Here's how the part is built. I have some questions about the finished solid (model axes, mm). Face numbers are marked on the shaded views. A direction names the side the tool comes from. Coordinates: 2 decimals unless noted, no trailing zeros. Write each loop counter-clockwise with the first axis right and the second up, starting at its lowest first coordinate (ties: lowest second). Pieces come first, ordered by that corner, then holes. Notation, with made-up numbers: (58.25, -15) - (100.25, -15) arc R34 ccw to (100.25, 17) - close; hole circle Ø11 at (10.5, 59). An arc over 180 degrees is marked (long way). Answer in a Markdown table with one row per item. Add a question column.
Item 1: Imagine slicing it at D-D (z = -7.62). Please give me the cut outline in (x, y).
Item 2: We'd pull the mould along Y, two halves only. Please class the marked faces 1, 2, 3 and 4: +Y half, -Y half, draft (parallel to the pull), parting line (faces both ways), or undercut.
Item 3: Imagine slicing it at B-B (y = 17.25). Please give me the cut outline in (x, z), plus the area to 3 significant figures.
Item 4: I'm going to push flat-ended pins straight in: pin 1 (4 mm diameter, centred on y = 20.5, z = -2.5, fed in from -X); pin 2 (3.5 mm diameter, centred on y = 13.5, z = -3.5, fed in from +X); pin 3 (2 mm diameter, centred on y = 4.5, z = -8.5, fed in from +X). Where does each tip first touch, or does it pass through?
Item 5: Which directions (+Z, -Z, +X, -X, +Y, -Y) give clear straight access to the entire face, cutting with the end or side of a thin tool? Please do the marked faces 5, 6 and 7.
Item 6: If I drill on probe 1 along Y at (x, z) = (-22.5, -8.5); probe 2 along X at (y, z) = (10, -11.5); probe 3 along Y at (x, z) = (-20.5, -7.25), over which ranges is the centre line in solid material (lowest first)? Write a range as from..to.
Item 7: Imagine slicing it at A-A (z = -4.5). Please give me the cut outline in (x, y).
Item 8: Imagine slicing it at C-C (x = -32.5). Please give me the cut outline in (y, z).
Autodesk Inventor part; units mm, degrees
ref_plane "YZ Plane" through (0, 0, 0) normal (1, 0, 0) x (0, 1, 0)
ref_plane "XZ Plane" through (0, 0, 0) normal (0, 1, 0) x (-1, 0, 0)
ref_plane "XY Plane" through (0, 0, 0) normal (0, 0, 1) x (1, 0, 0)
sketch "Sketch1" plane through (0, 0, 0) normal (0, 0, 1) x (1, 0, 0)
  line L0 (-18.3846, 28.5) -> (-18.3846, 22)
  line L1 (-18.3846, 22) -> (-22.3846, 18)
  line L2 (-22.3846, 18) -> (-22.3846, 7)
  line L3 (-22.3846, 7) -> (-18.3846, 3)
  line L4 (-18.3846, 3) -> (-18.3846, -3.5)
  line L5 (-18.3846, 28.5) -> (-31.1346, 28.5)
  line L6 (-31.1346, 28.5) -> (-31.1346, -3.5)
  line L7 (-31.1346, -3.5) -> (-18.3846, -3.5)
  line L8 (-22.3846, 7) -> (-23.3846, 7)
  line L9 (-23.3846, 7) -> (-23.3846, 18)
  line L10 (-23.3846, 18) -> (-22.3846, 18)
  line L11 (-31.1346, 11.0301) -> (-37.4846, 11.0301) construction
  point P0 (0, 0)
  dimension "d0" = 1
  dimension "d1" = 6.35
  dimension "d2" = 8.75
  dimension "d13" = 135
  dimension "d14" = 135
  dimension "d15" = 11
  dimension "d16" = 12.75
  dimension "d17" = 32
extrude "Extrusion1" add sketch "Sketch1" against normal blind 12 contours L0 L1 L10 L9 L8 L3 L4 L7 L6 L5
sketch "Sketch3" plane through (-31.1346, -3.5, 0) normal (-1, 0, 0) x (0, 0, 1)
  line L0 (0, 32) -> (0, 0)
  line L1 (0, 32) -> (-12, 32)
  line L2 (-12, 0) -> (-12, 32)
  line L3 (0, 0) -> (-12, 0)
  circle A0 centre (-7.62, 11.25) radius 1.27
  circle A1 centre (-7.62, 20.75) radius 1.27
  line L4 (-12, 21.5) -> (-12, 10.5) construction
  line L5 (-12, 16) -> (0, 16) construction
  point P0 (0, 3.5)
  dimension "d8" = 2.54
  dimension "d9" = 9.5
  dimension "d10" = 7.62
extrude "Extrusion3" add sketch "Sketch3" along normal blind 5 contours A0 | A1
properties part number "Limit Adapter"
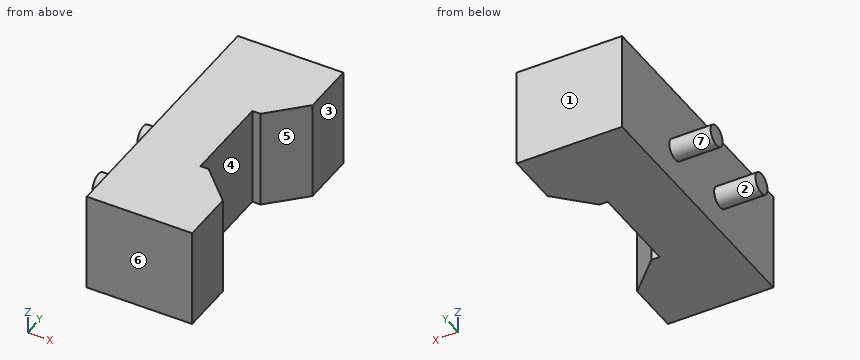
Here are the results:
| question | item | result |
|---|---|---|
| 1 | outline | (-36.13, 6.48) - (-31.13, 6.48) - (-31.13, -3.5) - (-18.38, -3.5) - (-18.38, 3) - (-22.38, 7) - (-23.38, 7) - (-23.38, 18) - (-22.38, 18) - (-18.38, 22) - (-18.38, 28.5) - (-31.13, 28.5) - (-31.13, 18.52) - (-36.13, 18.52) - (-36.13, 15.98) - (-31.13, 15.98) - (-31.13, 9.02) - (-36.13, 9.02) - close |
| 2 | face 1 | +Y half |
| 2 | face 2 | undercut |
| 2 | face 3 | draft |
| 2 | face 4 | undercut |
| 3 | outline | (-36.13, -8.89) - (-31.13, -8.89) - (-31.13, -12) - (-23.38, -12) - (-23.38, 0) - (-31.13, 0) - (-31.13, -6.35) - (-36.13, -6.35) - close |
| 3 | area | 106 mm2 |
| 4 | pin 1 | stops at x = -31.13 |
| 4 | pin 2 | stops at x = -23.38 |
| 4 | pin 3 | stops at x = -18.88 |
| 5 | face 5 | +Z, -Z, +X |
| 5 | face 6 | +Z, -Z, +X, -X, -Y |
| 5 | face 7 | -X |
| 6 | probe 1 | y = -3.5..7, 18..28.5 |
| 6 | probe 2 | x = -31.13..-23.38 |
| 6 | probe 3 | y = -3.5..5.12, 19.88..28.5 |
| 7 | outline | (-31.13, -3.5) - (-18.38, -3.5) - (-18.38, 3) - (-22.38, 7) - (-23.38, 7) - (-23.38, 18) - (-22.38, 18) - (-18.38, 22) - (-18.38, 28.5) - (-31.13, 28.5) - close |
| 8 | outline | circle Ø2.54 at (7.75, -7.62); circle Ø2.54 at (17.25, -7.62) |
